from build123d import *

# Parameters (mm, degrees)
F1_DEPTH = 101.6
F3_DEPTH = 38.1
F5_DEPTH = 25.4


with BuildPart() as f1:
    # F0 (on Front) → F1 (new body, symmetric)
    with BuildSketch(Plane.XZ):
        Polygon((0, 25.4), (0, 0), (127, 0), (177.8, 50.8), (228.6, 0), (254, 25.4), (128.276414, 151.123586), (102.876414, 125.723586), (152.4, 76.2), (101.6, 25.4), align=None)
    extrude(amount=F1_DEPTH, both=True)

    # F2 (on face) → F3 (cut)
    with BuildSketch(Plane(origin=(139.7, 0, 139.7), x_dir=(0, 1, 0), z_dir=(0.707107, 0, 0.707107))):
        with BuildLine():
            Line((50.8, 3.45539), (-50.8, 3.45539))
            ThreePointArc((-50.8, 3.45539), (-69.85, -15.59461), (-50.8, -34.64461))
            Line((-50.8, -34.64461), (50.8, -34.64461))
            ThreePointArc((50.8, -34.64461), (69.85, -15.59461), (50.8, 3.45539))
        make_face()
        with BuildLine():
            ThreePointArc((-50.8, -110.84461), (-69.85, -129.89461), (-50.8, -148.94461))
            Line((-50.8, -148.94461), (50.8, -148.94461))
            ThreePointArc((50.8, -148.94461), (69.85, -129.89461), (50.8, -110.84461))
            Line((50.8, -110.84461), (-50.8, -110.84461))
        make_face()
    extrude(amount=-F3_DEPTH, mode=Mode.SUBTRACT)

    # F4 (on face) → F5 (cut)
    with BuildSketch(Plane.XY.offset(25.4)):
        with BuildLine():
            Line((0, -25.4), (50.8, -25.4))
            ThreePointArc((50.8, -25.4), (76.2, 0), (50.8, 25.4))
            Line((50.8, 25.4), (0, 25.4))
            Line((0, 25.4), (0, -25.4))
        make_face()
    extrude(amount=-F5_DEPTH, mode=Mode.SUBTRACT)


solid = f1.part
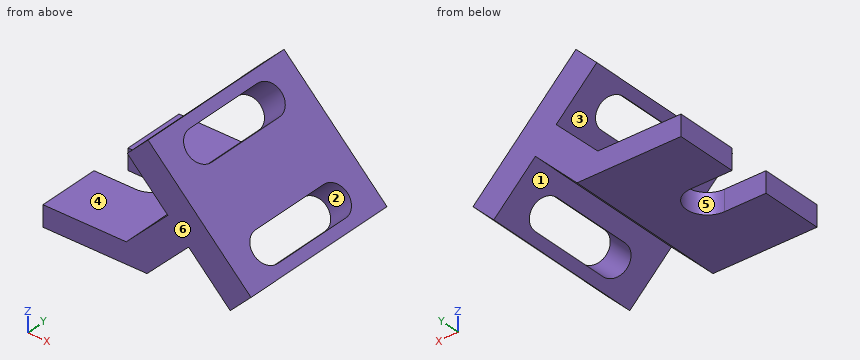
CAD build for the part. Positions are in the model's coordinates, mm. Face numbers are marked on the shaded views. A direction names the side the tool comes from. Coordinates: 2 decimals unless noted, no trailing zeros. Loops run counter-clockwise (first coordinate to the right, second up) from the corner with the lowest first, then second, coordinate; pieces in that order, holes last. Notation, with made-up numbers: (57, 62.5) -> (98, 62.5) arc R19 ccw to (98, 72.5) -> close; hole circle Ø10 at (-23.75, 72.5). An arc over 180 degrees is marked (long way). One line per item, written item: value.
1. Slice it at B-B on x = 44. Write the cut outline in (y, z).
Answers:
outline: (-101.6, 0) -> (-25.4, 0) -> (-25.4, 25.4) -> (-101.6, 25.4) -> close; (25.4, 0) -> (101.6, 0) -> (101.6, 25.4) -> (25.4, 25.4) -> close
2. Which spindle directions (+Z, -Z, +X, -X, +Y, -Y) get a long thin tool onto all of the face, cutting with end or side? Do the marked faces 1, 2 and 3. Say none if no direction does.
Answers:
face 1: -Z, +Y, -Y
face 2: none
face 3: -X, +Y, -Y
3. Pull direction Y, two halves, no side cores. Call the marked faces 4, 5 and 6: pulls with the +Y half, pulls with the -Y half, needs draft (parallel to the pull), parting line crosses it, or undercut.
Answers:
face 4: needs draft
face 5: undercut
face 6: pulls with the -Y half
4. Flat gauge pins, fed straight in: P1, Ø1.5, axis at y = 75.5, z = 38, coming from the +X side; P2, Ø3, axis at y = 21.5, z = 54, coming from the -X side; P3, Ø12, axis at y = 16, z = 79.5, coming from the -X side. Where does each tip first touch, or does it go through?
Answers:
P1: stops at x = 242.15
P2: stops at x = 128.7
P3: stops at x = 143.1
5. Drill centre lines: line 1 (Z direction, x = 74.5, y = 79.5); line 2 (Z direction, x = 125.5, y = -58); line 3 (X direction, y = 61.5, z = 56). Where is each one in solid material? Low to high. Write a range as [from, to].
Answers:
line 1: z = [0, 25.4]
line 2: z = [0, 49.3], [128.39, 148.35]
line 3: x = [132.2, 217.41]
6. Slice it at C-C on y = -87.5. Write the cut outline in (x, z).
Answers:
outline: (0, 0) -> (127, 0) -> (177.8, 50.8) -> (228.6, 0) -> (254, 25.4) -> (128.28, 151.12) -> (102.88, 125.72) -> (152.4, 76.2) -> (101.6, 25.4) -> (0, 25.4) -> close
7. Slice it at D-D on x = 169. Write the cut outline in (y, z).
Answers:
outline: (-101.6, 42) -> (101.6, 42) -> (101.6, 110.4) -> (-101.6, 110.4) -> close
8. Slice it at A-A on y = 43. Write the cut outline in (x, z), and give its area (3 significant figures).
Answers:
outline: (0, 0) -> (127, 0) -> (177.8, 50.8) -> (192.68, 35.92) -> (218.08, 61.32) -> (164.2, 115.2) -> (138.8, 89.8) -> (152.4, 76.2) -> (101.6, 25.4) -> (0, 25.4) -> close; (102.88, 125.72) -> (111.86, 116.74) -> (137.26, 142.14) -> (128.28, 151.12) -> close; (219.62, 8.98) -> (228.6, 0) -> (254, 25.4) -> (245.02, 34.38) -> close
area: 9,130 mm^2
